from build123d import *

# Parameters (mm, degrees)
F0_R     = 3.625
F1_DEPTH = 2.75
F2_R     = 0.5
F4_DEPTH = 1.5


with BuildPart() as f1:
    # F0 (on Right) → F1 (new body, symmetric)
    with BuildSketch(Plane.YZ):
        Circle(F0_R)
    extrude(amount=F1_DEPTH, both=True)

    # F2
    f2_edges = [f1.edges().sort_by_distance(p)[0] for p in [
        (2.75, -3.625, 0),
    ]]
    fillet(f2_edges, radius=F2_R)

    # F3 (on face) → F4 (join)
    with BuildSketch(Plane(origin=(-2.75, 0, 0), x_dir=(0, -1, 0), z_dir=(-1, 0, 0))):
        with BuildLine():
            Line((3.546565, -0.75), (5.046565, -0.75))
            Line((5.046565, -0.75), (5.046565, 0.75))
            Line((5.046565, 0.75), (3.546565, 0.75))
            ThreePointArc((3.546565, 0.75), (3.625, 0), (3.546565, -0.75))
        make_face()
        with BuildLine():
            Line((-3.546565, 0.75), (-5.046565, 0.75))
            Line((-5.046565, 0.75), (-5.046565, -0.75))
            Line((-5.046565, -0.75), (-3.546565, -0.75))
            ThreePointArc((-3.546565, -0.75), (-3.625, 0), (-3.546565, 0.75))
        make_face()
    extrude(amount=-F4_DEPTH)


solid = f1.part
Build history of the part. All positions in model axes, mm. A direction names the side the tool comes from. Give positions to 0.01 mm unless a question says otherwise; leave off trailing zeros. Order: outer loops, then holes, each group sorted by start corner. A loop starts at its lowest first (then second) coordinate and runs counter-clockwise, first axis right, second up. Notation, with made-up numbers: M 79.25,6 L 88.25,6 A37 cw 88.25,43 Z; hole C 32,76.25 d10. An arc over 180 degrees is marked long. Use one line per item in the form item = value.
Q1. Which spindle directions (+Z, -Z, +X, -X, +Y, -Y) get a long thin tool onto all of the face, cutting with end or side? Do faces 1 (the flat face through (-2, -4, 0.75)), 2 (the flat face through (-2, 4, -0.75)), 3 (the flat face through (-2, 4, 0.75)). Say none if no direction does.
Conclusion:
face_1 = +Z, +X, -X, -Y
face_2 = -Z, +X, -X, +Y
face_3 = +Z, +X, -X, +Y
Q2. Pin check, flat tips, straight feed: P1, Ø1.6, axis at x = -1.5, y = -4.5, coming from the -Z side; P2, Ø1.2, axis at y = 4, z = -0.5, coming from the +X side; P3, Ø1.2, axis at y = -4.5, z = -0.5, coming from the +X side. Stop position of each tip, or through.
Conclusion:
P1 = -0.75
P2 = 2.65
P3 = -1.25
Q3. Slice it at B-B, the plane x = 0.55. Write the cut outline in (y, z) (3 decimals), and give its area (3 significant figures).
Conclusion:
outline = C 0,0 d7.25
area = 41.3 mm2
Q4. Slice it at C-C, the plane y = 4. Write the cut outline in (x, z).
Conclusion:
outline = M -2.75,-0.75 L -1.25,-0.75 L -1.25,0.75 L -2.75,0.75 Z
Q5. Slice it at A-A, the plane z = 0. Write the cut outline in (x, y) (3 decimals), and give its area (3 significant figures).
Conclusion:
outline = M -2.75,-5.047 L -1.25,-5.047 L -1.25,-3.625 L 2.25,-3.625 A0.5 ccw 2.75,-3.125 L 2.75,3.125 A0.5 ccw 2.25,3.625 L -1.25,3.625 L -1.25,5.047 L -2.75,5.047 Z
area = 44.0 mm2
Q6. Wall check: probe 1 along Y at (x, z) = (1.65, 3); probe 2 along Y at (x, z) = (2.35, 2.25); probe 3 along Z at (x, y) = (-0.1, 1.75). Give the ranges that are in metal, low to high.
Conclusion:
probe_1 = -2.03 to 2.03
probe_2 = -2.83 to 2.83
probe_3 = -3.17 to 3.17
